from build123d import *

# Parameters (mm, degrees)
CELL_BLOCK_SKETCH_W = 127.601132068
CELL_BLOCK_SKETCH_H = 233.675
BOSS_EXTRUDE1_DEPTH = 5
SKETCH3_W           = 16
SKETCH3_H           = 233.675
BOSS_EXTRUDE3_DEPTH = 5
SKETCH4_R           = 3.25
CUT_EXTRUDE3_DEPTH  = 5
SKETCH6_R           = 10.875
CUT_EXTRUDE4_DEPTH  = 5
BOSS_EXTRUDE4_DEPTH = 10
SKETCH8_W           = 143
SKETCH8_H           = 3.175
BOSS_EXTRUDE5_DEPTH = 5
SKETCH9_W           = 118
SKETCH9_H           = 7
BOSS_EXTRUDE6_DEPTH = 25


with BuildPart() as part:
    # Cell Block Sketch → Boss-Extrude1 (new body)
    with BuildSketch(Plane(origin=(0, 0, 0), x_dir=(1, 0, 0), z_dir=(0, 1, 0))):
        Rectangle(CELL_BLOCK_SKETCH_W, CELL_BLOCK_SKETCH_H)
    extrude(amount=BOSS_EXTRUDE1_DEPTH)

    # Sketch3 → Boss-Extrude3 (add)
    with BuildSketch(Plane(origin=(0, 0, 0), x_dir=(1, 0, 0), z_dir=(0, 1, 0))):
        with Locations((-71.800566034, 0)):
            Rectangle(SKETCH3_W, SKETCH3_H)
    boss_extrude3 = extrude(amount=BOSS_EXTRUDE3_DEPTH)

    # Mirror1: Boss-Extrude3 across plane
    add(boss_extrude3.mirror(Plane(origin=(0, 0, 0), x_dir=(0, 0, 1), z_dir=(1, 0, 0))))

    # Sketch4 → Cut-Extrude3 (cut)
    with BuildSketch(Plane(origin=(0, 5, 0), x_dir=(1, 0, 0), z_dir=(0, 1, 0))):
        with Locations(Location((-71.800566034, 0, 0), (0, 0, 270))):
            Circle(SKETCH4_R)
        with Locations(Location((-71.800566034, -42, 0), (0, 0, 270))):
            Circle(SKETCH4_R)
        with Locations(Location((-71.800566034, -84, 0), (0, 0, 270))):
            Circle(SKETCH4_R)
        with Locations(Location((-71.800566034, 42, 0), (0, 0, 270))):
            Circle(SKETCH4_R)
        with Locations(Location((-71.800566034, 84, 0), (0, 0, 270))):
            Circle(SKETCH4_R)
    cut_extrude3 = extrude(amount=-CUT_EXTRUDE3_DEPTH, mode=Mode.SUBTRACT)

    # Mirror2: Cut-Extrude3 across plane
    add(cut_extrude3.mirror(Plane(origin=(0, 0, 0), x_dir=(0, 0, 1), z_dir=(1, 0, 0))), mode=Mode.SUBTRACT)

    # Sketch6 → Cut-Extrude4 (cut)
    with BuildSketch(Plane(origin=(0, 5, 0), x_dir=(1, 0, 0), z_dir=(0, 1, 0))):
        with Locations(Location((-33.050283017, 82.6375, 0), (0, 0, 270))):
            Circle(SKETCH6_R)
        with Locations(Location((-52.925566034, 94.1125, 0), (0, 0, 270))):
            Circle(SKETCH6_R)
        with Locations(Location((-13.175, 94.1125, 0), (0, 0, 270))):
            Circle(SKETCH6_R)
        with Locations(Location((-52.925566034, 71.1625, 0), (0, 0, 270))):
            Circle(SKETCH6_R)
        with Locations(Location((-33.050283017, 59.6875, 0), (0, 0, 270))):
            Circle(SKETCH6_R)
        with Locations(Location((-13.175, 71.1625, 0), (0, 0, 270))):
            Circle(SKETCH6_R)
        with Locations(Location((-52.925566034, 48.2125, 0), (0, 0, 270))):
            Circle(SKETCH6_R)
        with Locations(Location((-33.050283017, 36.7375, 0), (0, 0, 270))):
            Circle(SKETCH6_R)
        with Locations(Location((-13.175, 48.2125, 0), (0, 0, 270))):
            Circle(SKETCH6_R)
        with Locations(Location((-52.925566034, 25.2625, 0), (0, 0, 270))):
            Circle(SKETCH6_R)
        with Locations(Location((-33.050283017, 13.7875, 0), (0, 0, 270))):
            Circle(SKETCH6_R)
        with Locations(Location((-13.175, 25.2625, 0), (0, 0, 270))):
            Circle(SKETCH6_R)
        with Locations(Location((-52.925566034, 2.3125, 0), (0, 0, 270))):
            Circle(SKETCH6_R)
        with Locations(Location((-33.050283017, -9.1625, 0), (0, 0, 270))):
            Circle(SKETCH6_R)
        with Locations(Location((-13.175, 2.3125, 0), (0, 0, 270))):
            Circle(SKETCH6_R)
        with Locations(Location((-52.925566034, -20.6375, 0), (0, 0, 270))):
            Circle(SKETCH6_R)
        with Locations(Location((-33.050283017, -32.1125, 0), (0, 0, 270))):
            Circle(SKETCH6_R)
        with Locations(Location((-13.175, -20.6375, 0), (0, 0, 270))):
            Circle(SKETCH6_R)
        with Locations(Location((-52.925566034, -43.5875, 0), (0, 0, 270))):
            Circle(SKETCH6_R)
        with Locations(Location((-33.050283017, -55.0625, 0), (0, 0, 270))):
            Circle(SKETCH6_R)
        with Locations(Location((-13.175, -43.5875, 0), (0, 0, 270))):
            Circle(SKETCH6_R)
        with Locations(Location((-52.925566034, -66.5375, 0), (0, 0, 270))):
            Circle(SKETCH6_R)
        with Locations(Location((-33.050283017, -78.0125, 0), (0, 0, 270))):
            Circle(SKETCH6_R)
        with Locations(Location((-13.175, -66.5375, 0), (0, 0, 270))):
            Circle(SKETCH6_R)
        with Locations(Location((-52.925566034, -89.4875, 0), (0, 0, 270))):
            Circle(SKETCH6_R)
        with Locations(Location((-33.050283017, -100.9625, 0), (0, 0, 270))):
            Circle(SKETCH6_R)
        with Locations(Location((-13.175, -89.4875, 0), (0, 0, 270))):
            Circle(SKETCH6_R)
        with Locations(Location((33.050283017, 94.1125, 0), (0, 0, 270))):
            Circle(SKETCH6_R)
        with Locations(Location((13.175, 82.6375, 0), (0, 0, 270))):
            Circle(SKETCH6_R)
        with Locations(Location((52.925566034, 82.6375, 0), (0, 0, 270))):
            Circle(SKETCH6_R)
        with Locations(Location((13.175, 59.6875, 0), (0, 0, 270))):
            Circle(SKETCH6_R)
        with Locations(Location((33.050283017, 71.1625, 0), (0, 0, 270))):
            Circle(SKETCH6_R)
        with Locations(Location((52.925566034, 59.6875, 0), (0, 0, 270))):
            Circle(SKETCH6_R)
        with Locations(Location((13.175, 36.7375, 0), (0, 0, 270))):
            Circle(SKETCH6_R)
        with Locations(Location((33.050283017, 48.2125, 0), (0, 0, 270))):
            Circle(SKETCH6_R)
        with Locations(Location((52.925566034, 36.7375, 0), (0, 0, 270))):
            Circle(SKETCH6_R)
        with Locations(Location((13.175, 13.7875, 0), (0, 0, 270))):
            Circle(SKETCH6_R)
        with Locations(Location((33.050283017, 25.2625, 0), (0, 0, 270))):
            Circle(SKETCH6_R)
        with Locations(Location((52.925566034, 13.7875, 0), (0, 0, 270))):
            Circle(SKETCH6_R)
        with Locations(Location((13.175, -9.1625, 0), (0, 0, 270))):
            Circle(SKETCH6_R)
        with Locations(Location((33.050283017, 2.3125, 0), (0, 0, 270))):
            Circle(SKETCH6_R)
        with Locations(Location((52.925566034, -9.1625, 0), (0, 0, 270))):
            Circle(SKETCH6_R)
        with Locations(Location((13.175, -32.1125, 0), (0, 0, 270))):
            Circle(SKETCH6_R)
        with Locations(Location((33.050283017, -20.6375, 0), (0, 0, 270))):
            Circle(SKETCH6_R)
        with Locations(Location((52.925566034, -32.1125, 0), (0, 0, 270))):
            Circle(SKETCH6_R)
        with Locations(Location((13.175, -55.0625, 0), (0, 0, 270))):
            Circle(SKETCH6_R)
        with Locations(Location((33.050283017, -43.5875, 0), (0, 0, 270))):
            Circle(SKETCH6_R)
        with Locations(Location((52.925566034, -55.0625, 0), (0, 0, 270))):
            Circle(SKETCH6_R)
        with Locations(Location((13.175, -78.0125, 0), (0, 0, 270))):
            Circle(SKETCH6_R)
        with Locations(Location((33.050283017, -66.5375, 0), (0, 0, 270))):
            Circle(SKETCH6_R)
        with Locations(Location((52.925566034, -78.0125, 0), (0, 0, 270))):
            Circle(SKETCH6_R)
        with Locations(Location((13.175, -100.9625, 0), (0, 0, 270))):
            Circle(SKETCH6_R)
        with Locations(Location((33.050283017, -89.4875, 0), (0, 0, 270))):
            Circle(SKETCH6_R)
        with Locations(Location((52.925566034, -100.9625, 0), (0, 0, 270))):
            Circle(SKETCH6_R)
    extrude(amount=-CUT_EXTRUDE4_DEPTH, mode=Mode.SUBTRACT)

    # Sketch7 → Boss-Extrude4 (add)
    with BuildSketch(Plane(origin=(0, 5, 0), x_dir=(1, 0, 0), z_dir=(0, 1, 0))):
        Polygon((-79.800566034, 116.8375), (-79.800566034, 110.4875), (79.800566034, 110.4875), (79.800566034, 116.8375), (71.5, 116.8375), (71.5, 113.6625), (-71.5, 113.6625), (-71.5, 116.8375), align=None)
    extrude(amount=BOSS_EXTRUDE4_DEPTH)

    # Sketch8 → Boss-Extrude5 (add)
    with BuildSketch(Plane(origin=(0, 5, 0), x_dir=(1, 0, 0), z_dir=(0, 1, 0))):
        with Locations((0, 115.25)):
            Rectangle(SKETCH8_W, SKETCH8_H)
    extrude(amount=BOSS_EXTRUDE5_DEPTH)

    # Sketch9 → Boss-Extrude6 (add)
    with BuildSketch(Plane(origin=(0, 0, -116.8375), x_dir=(-1, 0, 0), z_dir=(0, 0, -1))):
        with Locations((0, 3.5)):
            Rectangle(SKETCH9_W, SKETCH9_H)
    extrude(amount=BOSS_EXTRUDE6_DEPTH)


solid = part.part
Can you work these out from the model? Positions are in its coordinate system, mm. Coordinates: 2 decimals unless noted, no trailing zeros. Loops run counter-clockwise (first coordinate to the right, second up) from the corner with the lowest first, then second, coordinate; pieces in that order, holes last. Notation, with made-up numbers: (19, -19.5) - (25, -19.5) arc R17 ccw to (25, 3.5) - close; hole circle Ø5 at (26.5, -9). An arc over 180 degrees is marked (long way). Put each result on its own line as item: value. Start each with the question number.
Item 1: If we mould it in two halves opening along Z, with no side actions, what happens to faces 1 (the face through (1, 2, 116.838)), 2 (the face through (70.82, 2.54, -38.9)), 3 (the face through (1, 7, -129))? For each: +Z half, -Z half, draft (parallel to the pull), parting line (faces both ways), or undercut.
Item 2: If I drill on line 1 along Z through (x, y) = (-69.5, 4.75); line 2 along X through (y, z) = (3.75, 103); line 3 along Z through (x, y) = (12, 13.75), over which ranges is the centre line in solid material (lowest first)?
Item 3: Suppose I cut it at A-A (z = -67.5). Please give me the cut outline in (x, y).
Item 4: Suppose I cut it at C-C (z = 74.5). Please give me the cut outline in (x, y), and give its area (3 significant figures).
Item 5: For pin 1 (12.5 mm diameter, centred on x = 0, z = -126.5, fed in from +Y); pin 2 (1.6 mm diameter, centred on x = 14, z = -115.5, fed in from +Y); pin 3 (1 mm diameter, centred on x = 27, y = 6.5, fed in from +Z), each with a flat end and sliding along its axis, tell me the tip position at first contact or that it passes through.
Item 6: Suppose I cut it at B-B (x = -6.5). State how many separate pieces and enclosed holes the cut face has, and give its area (3 significant figures).
Here are the results:
1. face 1: +Z half
1. face 2: undercut
1. face 3: draft
2. line 1: -116.84 to -86.3, -81.7 to -44.3, -39.7 to -2.3, 2.3 to 39.7, 44.3 to 81.7, 86.3 to 116.84
2. line 2: -79.8 to -43.73, -22.37 to 2.49, 23.86 to 42.24, 63.61 to 79.8
2. line 3: -113.66 to -110.49
3. outline: (-79.8, 0) - (-63.17, 0) - (-63.17, 5) - (-79.8, 5) - close; (-42.69, 0) - (-40.62, 0) - (-40.62, 5) - (-42.69, 5) - close; (-25.49, 0) - (-23.41, 0) - (-23.41, 5) - (-25.49, 5) - close; (-2.94, 0) - (5.61, 0) - (5.61, 5) - (-2.94, 5) - close; (20.74, 0) - (22.81, 0) - (22.81, 5) - (20.74, 5) - close; (43.29, 0) - (45.36, 0) - (45.36, 5) - (43.29, 5) - close; (60.49, 0) - (79.8, 0) - (79.8, 5) - (60.49, 5) - close
4. outline: (-79.8, 0) - (-60.33, 0) - (-60.33, 5) - (-79.8, 5) - close; (-45.52, 0) - (-43.34, 0) - (-43.34, 5) - (-45.52, 5) - close; (-22.76, 0) - (-20.58, 0) - (-20.58, 5) - (-22.76, 5) - close; (-5.77, 0) - (2.88, 0) - (2.88, 5) - (-5.77, 5) - close; (23.47, 0) - (25.64, 0) - (25.64, 5) - (23.47, 5) - close; (40.46, 0) - (42.63, 0) - (42.63, 5) - (40.46, 5) - close; (63.22, 0) - (79.8, 0) - (79.8, 5) - (63.22, 5) - close
4. area: 267 mm²
5. pin 1: y = 7
5. pin 2: y = 10
5. pin 3: z = -110.49
6. separate pieces: 10
6. enclosed holes: 0
6. area: 618 mm²
